Read the model definition and answer for the solid it produces. Units are mm, in the model's axes. A direction names the side the tool comes from. Give positions to 0.01 mm unless a question says otherwise; leave off trailing zeros. Loops run counter-clockwise (first coordinate to the right, second up) from the corner with the lowest first, then second, coordinate; pieces in that order, holes last. Notation, with made-up numbers: (53.25, -24.75) - (71.25, -24.75) arc R18 ccw to (71.25, 4.25) - close; hole circle Ø9 at (70, 75). An arc over 180 degrees is marked (long way). Write item = value, one per line.
Autodesk Inventor part; units mm, degrees
ref_plane "YZ Plane" through (0, 0, 0) normal (1, 0, 0) x (0, 1, 0)
ref_plane "XZ Plane" through (0, 0, 0) normal (0, 1, 0) x (-1, 0, 0)
ref_plane "XY Plane" through (0, 0, 0) normal (0, 0, 1) x (1, 0, 0)
sketch "Sketch1" plane through (0, 0, 0) normal (0, 1, 0) x (-1, 0, 0)
  line L0 (0, 0) -> (35.179, 0)
  line L1 (35.179, 0) -> (35.179, -15.24)
  line L2 (35.179, -15.24) -> (0, -15.24)
  line L3 (0, -15.24) -> (0, 0)
  dimension "d0" = 35.179
  dimension "d1" = 15.24
extrude "Extrusion1" add sketch "Sketch1" along normal blind 29.21
ref_plane "Work Plane1" through (0, 24.765, 0) normal (0, 1, 0) x (1, 0, 0)
sketch "Sketch2" plane through (0, 24.765, 0) normal (0, 1, 0) x (1, 0, 0)
  line L0 (0, 0) -> (6.35, 0)
  line L1 (6.35, 0) -> (6.35, 15.24)
  line L2 (6.35, 15.24) -> (0, 15.24)
  line L3 (0, 15.24) -> (0, 0)
  line L4 (-35.179, 0) -> (0, 0)
  line L5 (-35.179, 0) -> (-41.529, 0)
  line L6 (-41.529, 0) -> (-41.529, 15.24)
  line L7 (-41.529, 15.24) -> (-35.179, 15.24)
  line L8 (-35.179, 15.24) -> (-35.179, 0)
  dimension "d5" = 6.35
  dimension "d6" = 6.35
extrude "Extrusion2" add sketch "Sketch2" against normal blind 2.032
sketch "Sketch3" plane through (0, 29.21, 0) normal (0, 1, 0) x (1, 0, 0)
  circle A0 centre (-27.3494, 7.62) radius 2.9655
  point P0 (0, 0)
  point P1 (-41.529, 0)
  point P2 (-41.529, 15.24)
  dimension "d10" = 5.9309
extrude "Extrusion3" add sketch "Sketch3" along normal blind 4.5212
properties part number "AssaultReaper500Servo"
1) A cutting plane is placed at C-C on x = -20. Determine the outline of the cut face in (y, z).
Output:
outline = (0, -15.24) - (29.21, -15.24) - (29.21, 0) - (0, 0) - close
2) A cutting plane is placed at B-B on y = 28. Determine the outline of the cut face in (x, z), then the cut area to 3 significant figures.
Output:
outline = (-35.18, -15.24) - (0, -15.24) - (0, 0) - (-35.18, 0) - close
area = 536 mm²
3) A cutting plane is placed at A-A on z = -12. Determine the outline of the cut face in (x, y) (3 decimals).
Output:
outline = (-41.529, 22.733) - (-35.179, 22.733) - (-35.179, 0) - (0, 0) - (0, 22.733) - (6.35, 22.733) - (6.35, 24.765) - (0, 24.765) - (0, 29.21) - (-35.179, 29.21) - (-35.179, 24.765) - (-41.529, 24.765) - close
4) Find the intervals of material crossed by probe 1 along X at (y, z) = (26, -3); probe 2 along Y at (x, z) = (-32.5, -13); probe 3 along Y at (x, z) = (-37, -2.5) (3 decimals), in increasing order.
Output:
probe_1 = -35.18 to 0
probe_2 = 0 to 29.21
probe_3 = 22.733 to 24.765
5) A tool of negligible diameter and unlimited length cuts with its end or side. For faces 1 (the face through (0, 27, -8)), 2 (the face through (-38, 24.765, -8)), 3 (the face through (-35.179, 11, -8)), from which of +Z, -Z, +X, -X, +Y, -Y can it reach the whole face along a straight path? Write none if from no direction.
Output:
face_1 = +Z, -Z, +X, +Y
face_2 = +Z, -Z, -X, +Y
face_3 = +Z, -Z, -X, -Y
6) Each of these flat-tipped pins is pushed along its axis until it touches: P1, Ø1.9, axis at x = 4.5, z = -6, coming from the -Y side; P2, Ø5, axis at y = 27.5, z = -10, coming from the +X side; P3, Ø7.5, axis at y = 16, z = -10, coming from the -X side. Where does it stop, or does it pass through?
Output:
P1 = 22.73
P2 = 0
P3 = -35.18
7) A cutting plane is placed at D-D on z = -7.62. Determine the outline of the cut face in (x, y) (3 decimals), then the cut area to 3 significant figures.
Output:
outline = (-41.529, 22.733) - (-35.179, 22.733) - (-35.179, 0) - (0, 0) - (0, 22.733) - (6.35, 22.733) - (6.35, 24.765) - (0, 24.765) - (0, 29.21) - (-24.384, 29.21) - (-24.384, 33.731) - (-30.315, 33.731) - (-30.315, 29.21) - (-35.179, 29.21) - (-35.179, 24.765) - (-41.529, 24.765) - close
area = 1,080 mm²
